```python
from build123d import *
from build123d.topology import SkipClean

# Parameters (mm, degrees)
SKETCH1_R           = 84.709
SKETCH1_R_2         = 79.375
BOSS_EXTRUDE1_DEPTH = 19.05
BOSS_EXTRUDE2_START = 33.02
BOSS_EXTRUDE2_DEPTH = 33.02
SKETCH2_W           = 3.81
SKETCH2_H           = 38.1
CUT_EXTRUDE1_DEPTH  = 125.264032455
CIRPATTERN1_COUNT   = 4
CHAMFER1_SIZE       = 13.462
CHAMFER1_SIZE_2     = 33.319619221


with BuildPart() as part:
    # Sketch1 → Boss-Extrude1 (new body)
    with BuildSketch(Plane.XY):
        with Locations(Location((0, 0, 0), (0, 0, 180))):
            Circle(SKETCH1_R)
        with Locations(Location((0, 0, 0), (0, 0, 180))):
            Circle(SKETCH1_R_2, mode=Mode.SUBTRACT)
    extrude(amount=BOSS_EXTRUDE1_DEPTH)

    # Sketch3 → Boss-Extrude2 (add)
    with SkipClean():  # the faces are left unmerged after this step: merging them gives an invalid solid
        with BuildSketch(Plane(origin=(0, 0, 0), x_dir=(-1, 0, 0), z_dir=(0, 0, -1)).offset(BOSS_EXTRUDE2_START)):
            with BuildLine():
                Line((-5.715, 79.168992668), (-5.715, 84.515995267))
                ThreePointArc((-5.715, 84.515995267), (0, 84.709), (5.715, 84.515995267))
                Line((5.715, 84.515995267), (5.715, 79.168992668))
                ThreePointArc((5.715, 79.168992668), (0, 79.375), (-5.715, 79.168992668))
            make_face()
            with BuildLine():
                Line((-5.715, -79.168992668), (-5.715, -84.515995267))
                ThreePointArc((-5.715, -84.515995267), (0, -84.709), (5.715, -84.515995267))
                Line((5.715, -84.515995267), (5.715, -79.168992668))
                ThreePointArc((5.715, -79.168992668), (0, -79.375), (-5.715, -79.168992668))
            make_face()
            with BuildLine():
                Line((79.168992668, -5.715), (84.515995267, -5.715))
                ThreePointArc((84.515995267, -5.715), (84.709, 0), (84.515995267, 5.715))
                Line((84.515995267, 5.715), (79.168992668, 5.715))
                ThreePointArc((79.168992668, 5.715), (79.375, 0), (79.168992668, -5.715))
            make_face()
            with BuildLine():
                Line((-79.168992668, 5.715), (-84.515995267, 5.715))
                ThreePointArc((-84.515995267, 5.715), (-84.709, 0), (-84.515995267, -5.715))
                Line((-84.515995267, -5.715), (-79.168992668, -5.715))
                ThreePointArc((-79.168992668, -5.715), (-79.375, 0), (-79.168992668, 5.715))
            make_face()
        extrude(amount=-BOSS_EXTRUDE2_DEPTH)

    # Sketch2 → Cut-Extrude1 (cut, through all)
    with SkipClean():  # the faces are left unmerged after this step: merging them gives an invalid solid
        with BuildSketch(Plane(origin=(0, 0, 0), x_dir=(1, 0, 0), z_dir=(0, 1, 0))):
            with Locations((0, 7.62)):
                Rectangle(SKETCH2_W, SKETCH2_H)
        cut_extrude1 = extrude(amount=-CUT_EXTRUDE1_DEPTH, mode=Mode.SUBTRACT)

    # CirPattern1: Cut-Extrude1 ×4 about axis
    with SkipClean():  # the faces are left unmerged after this step: merging them gives an invalid solid
        cirpattern1_axis = Axis((0, 0, 0), (0, 0, 1))
        for i in range(1, CIRPATTERN1_COUNT):
            add(cut_extrude1.rotate(cirpattern1_axis, i * 360 / CIRPATTERN1_COUNT), mode=Mode.SUBTRACT)

    # Chamfer1
    # the kernel refuses this chamfer: 33.319619221, 13.462 mm, written as the material it adds along each edge
    with BuildSketch(Plane(origin=(-5.715, 170.913401218, 0), x_dir=(-0.9961057015681392, 0, 0.08816706473193561), z_dir=(0, -1, 0))) as chamfer1_piece_1_section:
        Polygon((CHAMFER1_SIZE * 0.996105701568, CHAMFER1_SIZE * 0.0881670647319), (-CHAMFER1_SIZE_2 * 0.0881670647311, CHAMFER1_SIZE_2 * 0.996105701559), (0, 0), align=None)
    chamfer1_piece_1 = extrude(amount=178.141814502, mode=Mode.PRIVATE)
    chamfer1_piece_1 = chamfer1_piece_1 & Plane(origin=(0, 0, -11.191625659), x_dir=(-1, 0, 0), z_dir=(0, 0, -1)) * Cylinder(84.709, 490, mode=Mode.PRIVATE)
    chamfer1_piece_1 = chamfer1_piece_1 - Plane(origin=(0, 0, -11.191625659), x_dir=(-1, 0, 0), z_dir=(0, 0, -1)) * Cylinder(79.375, 490, mode=Mode.PRIVATE)
    chamfer1_piece_1 = split(chamfer1_piece_1, bisect_by=Plane(origin=(-9.949714127, 81.358468366, -33.02), z_dir=(0, 0, 1)), keep=Keep.TOP, mode=Mode.PRIVATE)
    add(chamfer1_piece_1)
    with BuildSketch(Plane(origin=(-170.913401218, 5.715, 0), x_dir=(1.3071407043529467e-14, 0.9961057015681392, 0.08816706473193561), z_dir=(1, 0, 0))) as chamfer1_piece_2_section:
        Polygon((CHAMFER1_SIZE * 0.996105701568, -CHAMFER1_SIZE * 0.0881670647319), (-CHAMFER1_SIZE_2 * 0.0881670647311, -CHAMFER1_SIZE_2 * 0.996105701559), (0, 0), align=None)
    chamfer1_piece_2 = extrude(amount=178.141814502, mode=Mode.PRIVATE)
    chamfer1_piece_2 = chamfer1_piece_2 & Plane(origin=(0, 0, -11.191625637), x_dir=(-1, 0, 0), z_dir=(0, 0, -1)) * Cylinder(84.709, 490, mode=Mode.PRIVATE)
    chamfer1_piece_2 = chamfer1_piece_2 - Plane(origin=(0, 0, -11.191625637), x_dir=(-1, 0, 0), z_dir=(0, 0, -1)) * Cylinder(79.375, 490, mode=Mode.PRIVATE)
    chamfer1_piece_2 = split(chamfer1_piece_2, bisect_by=Plane(origin=(-81.358468349, 9.949714129, -33.02), z_dir=(0, 0, 1)), keep=Keep.TOP, mode=Mode.PRIVATE)
    add(chamfer1_piece_2)
    with BuildSketch(Plane(origin=(5.715, -7.228413283, 0), x_dir=(0.9961057015681392, 0, 0.08816706473193561), z_dir=(0, 1, 0))) as chamfer1_piece_3_section:
        Polygon((CHAMFER1_SIZE * 0.996105701568, CHAMFER1_SIZE * 0.0881670647319), (-CHAMFER1_SIZE_2 * 0.0881670647311, CHAMFER1_SIZE_2 * 0.996105701559), (0, 0), align=None)
    chamfer1_piece_3 = extrude(amount=178.141814502, mode=Mode.PRIVATE)
    chamfer1_piece_3 = chamfer1_piece_3 & Plane(origin=(0, 0, -11.191625637), x_dir=(-1, 0, 0), z_dir=(0, 0, -1)) * Cylinder(84.709, 490, mode=Mode.PRIVATE)
    chamfer1_piece_3 = chamfer1_piece_3 - Plane(origin=(0, 0, -11.191625637), x_dir=(-1, 0, 0), z_dir=(0, 0, -1)) * Cylinder(79.375, 490, mode=Mode.PRIVATE)
    chamfer1_piece_3 = split(chamfer1_piece_3, bisect_by=Plane(origin=(9.949714129, 81.358468349, -33.02), z_dir=(0, 0, 1)), keep=Keep.TOP, mode=Mode.PRIVATE)
    add(chamfer1_piece_3)
    with BuildSketch(Plane(origin=(-7.228413283, 5.715, 0), x_dir=(-1.3071407043529467e-14, 0.9961057015681392, 0.08816706473193563), z_dir=(1, 0, 0))) as chamfer1_piece_4_section:
        Polygon((CHAMFER1_SIZE * 0.996105701568, -CHAMFER1_SIZE * 0.0881670647319), (-CHAMFER1_SIZE_2 * 0.0881670647311, -CHAMFER1_SIZE_2 * 0.996105701559), (0, 0), align=None)
    chamfer1_piece_4 = extrude(amount=178.141814502, mode=Mode.PRIVATE)
    chamfer1_piece_4 = chamfer1_piece_4 & Plane(origin=(0, 0, -11.191625658), x_dir=(-1, 0, 0), z_dir=(0, 0, -1)) * Cylinder(84.709, 490, mode=Mode.PRIVATE)
    chamfer1_piece_4 = chamfer1_piece_4 - Plane(origin=(0, 0, -11.191625658), x_dir=(-1, 0, 0), z_dir=(0, 0, -1)) * Cylinder(79.375, 490, mode=Mode.PRIVATE)
    chamfer1_piece_4 = split(chamfer1_piece_4, bisect_by=Plane(origin=(81.358468366, 9.949714127, -33.02), z_dir=(0, 0, 1)), keep=Keep.TOP, mode=Mode.PRIVATE)
    add(chamfer1_piece_4)
    with BuildSketch(Plane(origin=(-5.715, -170.913401218, 0), x_dir=(-0.9961057015681392, 0, 0.08816706473193561), z_dir=(0, 1, 0))) as chamfer1_piece_5_section:
        Polygon((CHAMFER1_SIZE * 0.996105701568, -CHAMFER1_SIZE * 0.0881670647319), (-CHAMFER1_SIZE_2 * 0.0881670647311, -CHAMFER1_SIZE_2 * 0.996105701559), (0, 0), align=None)
    chamfer1_piece_5 = extrude(amount=178.141814502, mode=Mode.PRIVATE)
    chamfer1_piece_5 = chamfer1_piece_5 & Plane(origin=(0, 0, -11.191625637), x_dir=(-1, 0, 0), z_dir=(0, 0, -1)) * Cylinder(84.709, 490, mode=Mode.PRIVATE)
    chamfer1_piece_5 = chamfer1_piece_5 - Plane(origin=(0, 0, -11.191625637), x_dir=(-1, 0, 0), z_dir=(0, 0, -1)) * Cylinder(79.375, 490, mode=Mode.PRIVATE)
    chamfer1_piece_5 = split(chamfer1_piece_5, bisect_by=Plane(origin=(-9.949714129, -81.358468349, -33.02), z_dir=(0, 0, 1)), keep=Keep.TOP, mode=Mode.PRIVATE)
    add(chamfer1_piece_5)
    with BuildSketch(Plane(origin=(7.228413283, -5.715, 0), x_dir=(-1.5553319773313542e-14, -0.9961057015681392, 0.08816706473193561), z_dir=(-1, 0, 0))) as chamfer1_piece_6_section:
        Polygon((CHAMFER1_SIZE * 0.996105701568, -CHAMFER1_SIZE * 0.0881670647319), (-CHAMFER1_SIZE_2 * 0.0881670647311, -CHAMFER1_SIZE_2 * 0.996105701559), (0, 0), align=None)
    chamfer1_piece_6 = extrude(amount=178.141814502, mode=Mode.PRIVATE)
    chamfer1_piece_6 = chamfer1_piece_6 & Plane(origin=(0, 0, -11.191625659), x_dir=(-1, 0, 0), z_dir=(0, 0, -1)) * Cylinder(84.709, 490, mode=Mode.PRIVATE)
    chamfer1_piece_6 = chamfer1_piece_6 - Plane(origin=(0, 0, -11.191625659), x_dir=(-1, 0, 0), z_dir=(0, 0, -1)) * Cylinder(79.375, 490, mode=Mode.PRIVATE)
    chamfer1_piece_6 = split(chamfer1_piece_6, bisect_by=Plane(origin=(-81.358468366, -9.949714127, -33.02), z_dir=(0, 0, 1)), keep=Keep.TOP, mode=Mode.PRIVATE)
    add(chamfer1_piece_6)
    with BuildSketch(Plane(origin=(5.715, 7.228413283, 0), x_dir=(0.9961057015681392, 0, 0.08816706473193563), z_dir=(0, -1, 0))) as chamfer1_piece_7_section:
        Polygon((CHAMFER1_SIZE * 0.996105701568, -CHAMFER1_SIZE * 0.0881670647319), (-CHAMFER1_SIZE_2 * 0.0881670647311, -CHAMFER1_SIZE_2 * 0.996105701559), (0, 0), align=None)
    chamfer1_piece_7 = extrude(amount=178.141814502, mode=Mode.PRIVATE)
    chamfer1_piece_7 = chamfer1_piece_7 & Plane(origin=(0, 0, -11.191625659), x_dir=(-1, 0, 0), z_dir=(0, 0, -1)) * Cylinder(84.709, 490, mode=Mode.PRIVATE)
    chamfer1_piece_7 = chamfer1_piece_7 - Plane(origin=(0, 0, -11.191625659), x_dir=(-1, 0, 0), z_dir=(0, 0, -1)) * Cylinder(79.375, 490, mode=Mode.PRIVATE)
    chamfer1_piece_7 = split(chamfer1_piece_7, bisect_by=Plane(origin=(9.949714127, -81.358468366, -33.02), z_dir=(0, 0, 1)), keep=Keep.TOP, mode=Mode.PRIVATE)
    add(chamfer1_piece_7)
    with BuildSketch(Plane(origin=(170.913401218, -5.715, 0), x_dir=(1.555331977331354e-14, -0.9961057015681392, 0.08816706473193561), z_dir=(-1, 0, 0))) as chamfer1_piece_8_section:
        Polygon((CHAMFER1_SIZE * 0.996105701568, -CHAMFER1_SIZE * 0.0881670647319), (-CHAMFER1_SIZE_2 * 0.0881670647311, -CHAMFER1_SIZE_2 * 0.996105701559), (0, 0), align=None)
    chamfer1_piece_8 = extrude(amount=178.141814502, mode=Mode.PRIVATE)
    chamfer1_piece_8 = chamfer1_piece_8 & Plane(origin=(0, 0, -11.191625637), x_dir=(-1, 0, 0), z_dir=(0, 0, -1)) * Cylinder(84.709, 490, mode=Mode.PRIVATE)
    chamfer1_piece_8 = chamfer1_piece_8 - Plane(origin=(0, 0, -11.191625637), x_dir=(-1, 0, 0), z_dir=(0, 0, -1)) * Cylinder(79.375, 490, mode=Mode.PRIVATE)
    chamfer1_piece_8 = split(chamfer1_piece_8, bisect_by=Plane(origin=(81.358468349, -9.949714129, -33.02), z_dir=(0, 0, 1)), keep=Keep.TOP, mode=Mode.PRIVATE)
    add(chamfer1_piece_8)


solid = part.part
```
Work out the finished part from the listing and answer in its coordinate system (mm). A direction names the side the tool comes from. Give positions to 0.01 mm unless a question says otherwise; leave off trailing zeros. Order: outer loops, then holes, each group sorted by start corner. A loop starts at its lowest first (then second) coordinate and runs counter-clockwise, first axis right, second up. Notation, with made-up numbers: M -5,61 L 18,61 A17 ccw 18,76 Z; hole C 85,71 d9. An arc over 180 degrees is marked long. Return JSON: item names as keys, results as strings.
1) Section C-C, the plane z = -20.5 is taken. Give the number of separate pieces and of enclosed holes in the cut face, plus the area to 3 significant figures.
Resolved:
{"separate pieces": "8", "enclosed holes": "0", "area": "385 mm^2"}
2) A tool of negligible diameter and unlimited length cuts with its end or side. For faces 4 (the flat face through (12.6, -80.71, -16.28)), 5 (the flat face through (-82, -1.905, -7)), 6 (the flat face through (0, 82, 11.43)), from which of +Z, -Z, +X, -X, +Y, -Y can it reach the whole face along a straight path? Write none if from no direction.
Resolved:
{"face 4": "-Z, +X, +Y, -Y", "face 5": "+X, -X", "face 6": "+Y, -Y"}
3) For a pull along Z with two mould halves and no side action, classify faces 1 (the flat face through (-1.905, -82, -7)), 2 (the flat face through (76, 25, 19.05)), 3 (the flat face through (0, -82, -33.02)) as +Z half, -Z half, draft (parallel to the pull), parting line (faces both ways), or undercut.
Resolved:
{"face 1": "undercut", "face 2": "+Z half", "face 3": "-Z half"}
4) Section A-A, the plane x = -25.5 is taken. Write down the section's boundary in (y, z), plus the area to 3 significant figures.
Resolved:
{"outline": "M -80.78,0 L -75.17,0 L -75.17,19.05 L -80.78,19.05 Z; M 75.17,0 L 80.78,0 L 80.78,19.05 L 75.17,19.05 Z", "area": "214 mm^2"}
5) Section B-B, the plane y = -30 is taken. Write down the section's boundary in (x, z), plus the area to 3 significant figures.
Resolved:
{"outline": "M -79.22,0 L -73.49,0 L -73.49,19.05 L -79.22,19.05 Z; M 73.49,0 L 79.22,0 L 79.22,19.05 L 73.49,19.05 Z", "area": "218 mm^2"}
6) Each of these flat-tipped pins is pushed along its axis until it touches: pin 1 (6 mm diameter, centred on x = -83, z = -12, fed in from +Y); pin 2 (5 mm diameter, centred on x = 3, z = 3.5, fed in from +Y); pin 3 (1.5 mm diameter, centred on y = -13, z = -7.5, fed in from +X). Where does it stop, or does it pass through?
Resolved:
{"pin 1": "y = 15.54", "pin 2": "y = 84.69", "pin 3": "x = 83.82"}
7) Straight lines are drawn through the part: line 1 along Y through (x, z) = (-0.5, 12); line 2 along Y through (x, z) = (19, 12). For each, find the intervals that lie inside material, in ascending order. Write a range as [from, to].
Resolved:
{"line 1": "[-84.71, -79.37], [79.37, 84.71]", "line 2": "[-82.55, -77.07], [77.07, 82.55]"}
